The figure shows three views and two pictorial views of one solid part (mm, origin at its lowest corner). Answer the questions. A direction names the side the tool comes from. Round coordinates to 2 decimals unless told otherwise and drop trailing zeros. Order: outer loops, then holes, each group sorted by start corner. A loop starts at its lowest first (then second) coordinate and runs counter-clockwise, first axis right, second up.
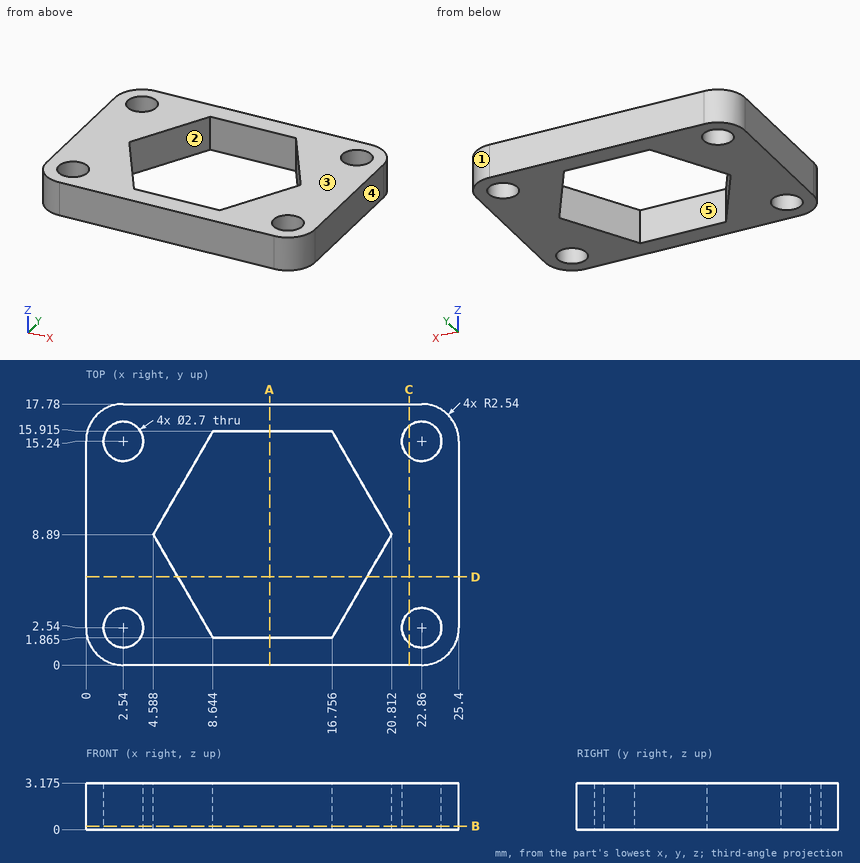
Item 1: Find section C-C (x = 22). Write down the section's boundary in (y, z) (1 decimal).
Item 2: Given pin 1 (1.6 mm diameter, centred on x = 2.54, y = 2.54, fed in from -Z), flat-ended and moving along its own axis, determine where the tip first touches the part or whether it passes through.
Item 3: Find the intervals of material crossed by line 1 along Y through (x, z) = (22.86, 1.05); line 2 along X through (y, z) = (15.24, 1.8) (1 decimal); line 3 along Y through (x, z) = (15.75, 0.95) (3 decimals), in increasing order.
Item 4: Find section A-A (x = 12.5). Write down the section's boundary in (y, z) (3 decimals).
Item 5: For a pull along X with two mould halves and no side action, classify the marked faces 1, 2 and 3 as released by +X, released by -X, zero draft, split by the parting line, or undercut.
Item 6: Find section D-D (y = 6). Write down the section's boundary in (x, z) (1 decimal).
Item 7: Find section B-B (z = 0.25). State how many separate pieces and enclosed holes the cut face has, plus the area to 3 significant figures.
Item 8: A tool of negligible diameter and unlimited length cuts with its end or side. For the marked faces 4 and 5, from which of +Z, -Z, +X, -X, +Y, -Y can it reach the whole face along a straight path? Write none if from no direction.
Model answer:
1. outline: (0, 0) - (1.5, 0) - (1.5, 3.2) - (0, 3.2) - close; (3.6, 0) - (14.2, 0) - (14.2, 3.2) - (3.6, 3.2) - close; (16.3, 0) - (17.8, 0) - (17.8, 3.2) - (16.3, 3.2) - close
2. pin 1: passes through
3. line 1: y = 0 to 1.19, 3.89 to 13.89, 16.59 to 17.78
3. line 2: x = 0 to 1.2, 3.9 to 8.3, 17.1 to 21.5, 24.2 to 25.4
3. line 3: y = 0 to 1.865, 15.915 to 17.78
4. outline: (0, 0) - (1.865, 0) - (1.865, 3.175) - (0, 3.175) - close; (15.915, 0) - (17.78, 0) - (17.78, 3.175) - (15.915, 3.175) - close
5. face 1: released by +X
5. face 2: undercut
5. face 3: zero draft
6. outline: (0, 0) - (6.3, 0) - (6.3, 3.2) - (0, 3.2) - close; (19.1, 0) - (25.4, 0) - (25.4, 3.2) - (19.1, 3.2) - close
7. separate pieces: 1
7. enclosed holes: 5
7. area: 252 mm2
8. face 4: +Z, -Z, +X, +Y, -Y
8. face 5: +Z, -Z
